Design review of the part built by this model. Coordinates are the model's own, in mm. Face numbers are marked on the shaded views. A direction names the side the tool comes from. Round coordinates to 2 decimals unless told otherwise and drop trailing zeros. Order: outer loops, then holes, each group sorted by start corner. A loop starts at its lowest first (then second) coordinate and runs counter-clockwise, first axis right, second up.
from build123d import *

# Parameters (mm, degrees)
SKETCH_1_R          = 5
SKETCH_1_R_2        = 4.5
EXTRUDE_1_DEPTH     = 1
SKETCH_1_5_R        = 4.5
SKETCH_1_5_R_2      = 4
EXTRUDE_2_DEPTH     = 2
SKETCH_1_6_R        = 4
SKETCH_1_6_W        = 5
SKETCH_1_6_H        = 5
EXTRUDE_3_DEPTH     = 10.5
SKETCH_1_7_W        = 5
SKETCH_1_7_H        = 5
EXTRUDE_4_DEPTH     = 18.5
CUT_EXTRUDE_1_DEPTH = 1
SKETCH_5_R          = 1.65
CUT_EXTRUDE_2_DEPTH = 10
FILLET_1_R          = 1
CHAMFER_1_SIZE      = 0.3


with BuildPart() as part:
    # Sketch 1 → Extrude 1 (new body)
    with BuildSketch(Plane(origin=(0, 0, 0), x_dir=(1, 0, 0), z_dir=(0, 1, 0))):
        with Locations(Location((0, 0, 0), (0, 0, 270))):
            Circle(SKETCH_1_R)
        with Locations(Location((0, 0, 0), (0, 0, 270))):
            Circle(SKETCH_1_R_2, mode=Mode.SUBTRACT)
    extrude(amount=EXTRUDE_1_DEPTH)

    # Sketch 1_5 → Extrude 2 (add)
    with BuildSketch(Plane(origin=(0, 0, 0), x_dir=(1, 0, 0), z_dir=(0, 1, 0))):
        with Locations(Location((0, 0, 0), (0, 0, 270))):
            Circle(SKETCH_1_5_R)
        with Locations(Location((0, 0, 0), (0, 0, 270))):
            Circle(SKETCH_1_5_R_2, mode=Mode.SUBTRACT)
    extrude(amount=EXTRUDE_2_DEPTH)

    # Sketch 1_6 → Extrude 3 (add)
    # profile 1 of 2: a face of its own
    with BuildSketch(Plane(origin=(0, 0, 0), x_dir=(1, 0, 0), z_dir=(0, 1, 0))):
        with Locations(Location((0, 0, 0), (0, 0, 90))):
            Circle(SKETCH_1_6_R)
        Rectangle(SKETCH_1_6_W, SKETCH_1_6_H, mode=Mode.SUBTRACT)
    # profile 2 of 2: a face of its own
    with BuildSketch(Plane(origin=(0, 0, 0), x_dir=(1, 0, 0), z_dir=(0, 1, 0))):
        Rectangle(SKETCH_1_6_W, SKETCH_1_6_H)
    extrude(amount=EXTRUDE_3_DEPTH)

    # Sketch 1_7 → Extrude 4 (add)
    with BuildSketch(Plane(origin=(0, 0, 0), x_dir=(1, 0, 0), z_dir=(0, 1, 0))):
        Rectangle(SKETCH_1_7_W, SKETCH_1_7_H)
    extrude(amount=EXTRUDE_4_DEPTH)

    # Sketch 3 → Cut-Extrude 1 (cut)
    with BuildSketch(Plane.XZ):
        with BuildLine():
            Line((1, 1), (1, -1))
            ThreePointArc((1, -1), (0, -2), (-1, -1))
            Line((-1, -1), (-1, 1))
            ThreePointArc((-1, 1), (0, 2), (1, 1))
        make_face()
    extrude(amount=-CUT_EXTRUDE_1_DEPTH, mode=Mode.SUBTRACT)

    # Sketch 4 → Cut-Revolve 1 (revolve, cut)
    with BuildSketch(Plane.XY, mode=Mode.PRIVATE) as cut_revolve_1_sk:
        Polygon((0, 8.5), (-1.65, 8.5), (0, 7.816547622), align=None)
    revolve(cut_revolve_1_sk.sketch.rotate(Axis((0, -0.586194708, 0), (0, 1, 0)), 90), axis=Axis((0, -0.586194708, 0), (0, 1, 0)), mode=Mode.SUBTRACT)

    # Sketch 5 → Cut-Extrude 2 (cut)
    with BuildSketch(Plane(origin=(0, 18.5, 0), x_dir=(1, 0, 0), z_dir=(0, 1, 0))):
        with Locations(Location((0, 0, 0), (0, 0, 270))):
            Circle(SKETCH_5_R)
    extrude(amount=-CUT_EXTRUDE_2_DEPTH, mode=Mode.SUBTRACT)

    # Fillet 1
    fillet_1_edges = [part.edges().sort_by_distance(p)[0] for p in [
        (-2.5, 14.5, -2.5),
        (-2.5, 14.5, 2.5),
        (2.5, 14.5, 2.5),
        (2.5, 14.5, -2.5),
    ]]
    fillet(fillet_1_edges, radius=FILLET_1_R)

    # Chamfer 1
    chamfer_1_edges = [part.edges().sort_by_distance(p)[0] for p in [
        (0, 2, -4.5),
        (0, 1, -5),
        (0, 10.5, 4),
        (0, 0, -5),
        (0, 18.5, -1.65),
        (2.5, 18.5, 0),
        (0, 18.5, 2.5),
        (-2.5, 18.5, 0),
        (0, 18.5, -2.5),
        (-2.207106781, 18.5, -2.207106781),
        (-2.207106781, 18.5, 2.207106781),
        (2.207106781, 18.5, -2.207106781),
        (2.207106781, 18.5, 2.207106781),
    ]]
    chamfer(chamfer_1_edges, length=CHAMFER_1_SIZE)


solid = part.part
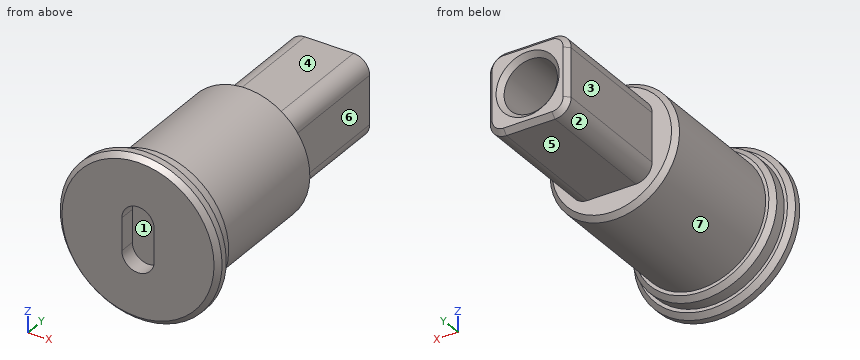
1) Take a section at B-B on y = 5. Give the boundary of the cut face in (x, z).
Results:
outline: circle Ø8 at (0, 0)
2) To check wall thickness, follow line 1 along X through (y, z) = (14, 0); line 2 along Y through (x, z) = (4, 0.5); line 3 along Y through (x, z) = (-1.25, 3.25). State the ranges of each line that lie inside material, in increasing order.
Results:
line 1: x = -2.5 to -1.65, 1.65 to 2.5
line 2: y = 0 to 2
line 3: y = 0 to 10.5
3) The part is to be moulded in two halves that separate along Z. For the marked faces 1, 2 and 3, say which applies: released by +Z, released by -Z, zero draft, split by the parting line, or undercut.
Results:
face 1: undercut
face 2: released by -Z
face 3: zero draft
4) Clearance check with flat-ended pins moving along their axes: P1, Ø2.5, axis at x = 0, y = 14, coming from the +Z side; P2, Ø1, axis at x = 0, y = 11.5, coming from the -Z side; P3, Ø2.5, axis at y = 13.5, z = -0.5, coming from the -X side; P4, Ø1, axis at x = 1, z = -3.5, coming from the -Y side. State where each tip first meets the part, or that it passes through.
Results:
P1: stops at z = 2.5
P2: stops at z = -2.5
P3: stops at x = -2.5
P4: stops at y = 0
5) For the marked faces 4, 5, 6 and 7, list the 3-axis set-ups (+Z, -Z, +X, -X, +Y, -Y) from which the entire face can be reached by the end or side of a thin tool; tool diameter is ignored.
Results:
face 4: +Z, +X, -X, +Y
face 5: -Z, +X, -X, +Y
face 6: +Z, -Z, +X, +Y
face 7: +Y
6) Take a section at C-C on y = 8.25. Give the boundary of the cut face in (x, z), plus the area to 3 significant figures.
Results:
outline: circle Ø8 at (0, 0); hole circle Ø2.09 at (0, 0)
area: 46.8 mm2
7) Take a section at A-A on y = 11.25. Give the boundary of the cut face in (x, z), plus the area to 3 significant figures.
Results:
outline: (-2.5, -1.5) arc R1 ccw to (-1.5, -2.5) - (1.5, -2.5) arc R1 ccw to (2.5, -1.5) - (2.5, 1.5) arc R1 ccw to (1.5, 2.5) - (-1.5, 2.5) arc R1 ccw to (-2.5, 1.5) - close; hole circle Ø3.3 at (0, 0)
area: 15.6 mm2
